Verification items for this drawing (mm, ordinates from the low corner). A direction names the side the tool comes from. Give positions to 0.01 mm unless a question says otherwise; leave off trailing zeros. Write each loop counter-clockwise with the first axis right and the second up, starting at its lowest first coordinate (ties: lowest second). Pieces come first, ordered by that corner, then holes. Notation, with made-up numbers: M 25.25,-12 L 83.25,-12 A20 ccw 83.25,12 Z; hole C 85.5,76.25 d3. An arc over 180 degrees is marked long. Use one line per item in the form item = value. Start each with the question number.
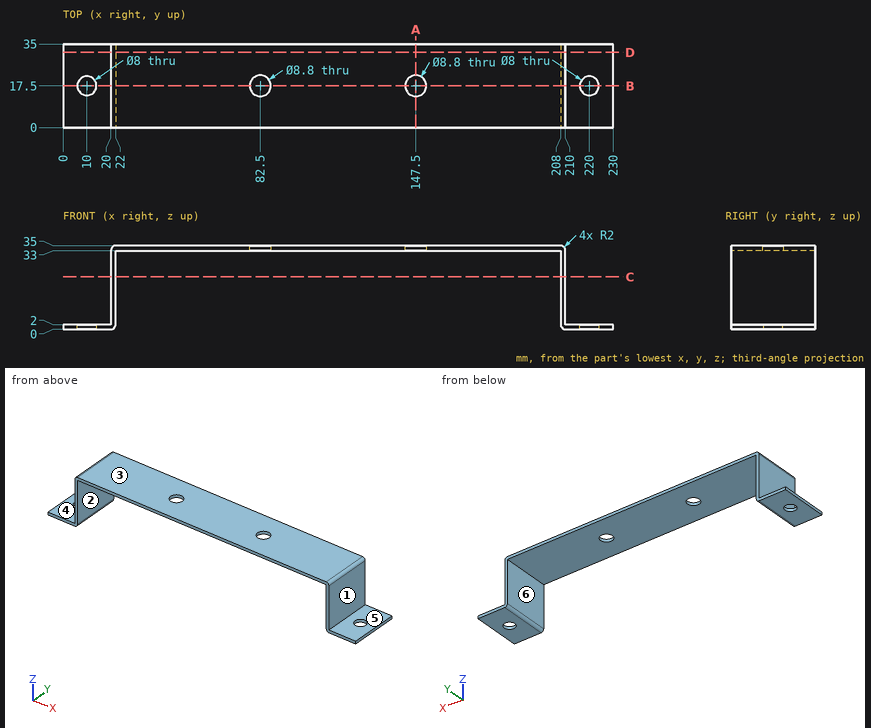
(1) Depth check by flat-ended pin: pin 1 (6 mm diameter, centred on y = 24.5, z = 11.5, fed in from +X); pin 2 (16 mm diameter, centred on x = 224.5, y = 11, fed in from +Z); pin 3 (2 mm diameter, centred on y = 26, z = 13, fed in from -X); pin 4 (7 mm diameter, centred on x = 10, y = 17.5, fed in from +Z). Enter the tip coordinate at first touch or a pass-through.
(2) Thickness scan on probe 1 along X at (y, z) = (23.5, 26.5); probe 2 along Y at (x, z) = (147.5, 33.8); probe 3 along Y at (x, z) = (10, 1). Record the ranges inside material, lowest first. Write a range as [from, to].
(3) Tool access check on the marked faces 4, 5 and 6. Record the directions out of +Z, -Z, +X, -X, +Y, -Y that give a thin tool (end or side, any length) a straight path to the whole face; none if there is none.
(4) Draft check along X on the marked faces 1, 2 and 3. Enter one of: released by +X, released by -X, zero draft, split by the parting line, or undercut.
(5) Sectioned sample at B-B, the plane y = 17.5. State how many separate pieces and enclosed holes the cut face has, plus the area to 3 significant figures.
(6) Sectioned sample at C-C, the plane z = 22. Record the boundary of the cut face in (x, y).
(7) Sectioned sample at A-A, the plane x = 147.5. Record the boundary of the cut face in (y, z).
(8) Sectioned sample at D-D, the plane y = 31.5. Record the boundary of the cut face in (x, z).
Numbers:
q1.pin_1 = 210
q1.pin_2 = 2
q1.pin_3 = 20
q1.pin_4 = through
q2.probe_1 = [20, 22], [208, 210]
q2.probe_2 = [0, 13.1], [21.9, 35]
q2.probe_3 = [0, 13.5], [21.5, 35]
q3.face_4 = +Z, -X, +Y, -Y
q3.face_5 = +Z, +X, +Y, -Y
q3.face_6 = -Z, +Y, -Y
q4.face_1 = released by +X
q4.face_2 = undercut
q4.face_3 = zero draft
q5.separate_pieces = 5
q5.enclosed_holes = 0
q5.area = 521 mm2
q6.outline = M 20,0 L 22,0 L 22,35 L 20,35 Z; M 208,0 L 210,0 L 210,35 L 208,35 Z
q7.outline = M 0,33 L 13.1,33 L 13.1,35 L 0,35 Z; M 21.9,33 L 35,33 L 35,35 L 21.9,35 Z
q8.outline = M 0,0 L 20,0 A2 ccw 22,2 L 22,33 L 208,33 L 208,2 A2 ccw 210,0 L 230,0 L 230,2 L 210,2 L 210,33 A2 ccw 208,35 L 22,35 A2 ccw 20,33 L 20,2 L 0,2 Z
